```python
from build123d import *

# Parameters (mm, degrees)
SKETCH1_W           = 96.52
SKETCH1_H           = 44.45
BOSS_EXTRUDE1_DEPTH = 6.096
CUT_EXTRUDE1_REACH  = 108.961
SKETCH2_R           = 11.50874
CUT_EXTRUDE2_REACH  = 108.438
SKETCH3_R           = 3.3782
CUT_EXTRUDE3_REACH  = 108.961
SKETCH7_W           = 12.7635
SKETCH7_H           = 12.192
CUT_EXTRUDE5_DEPTH  = 104.946532487
FILLET1_R           = 11.43


with BuildPart() as part:
    # Sketch1 → Boss-Extrude1 (new, symmetric)
    with BuildSketch(Plane.XY):
        with Locations((48.26, -22.225)):
            Rectangle(SKETCH1_W, SKETCH1_H)
    extrude(amount=BOSS_EXTRUDE1_DEPTH, both=True)

    # Sketch2 → Cut-Extrude1 (cut, up to next)
    with BuildSketch(Plane.XY.offset(6.096), mode=Mode.PRIVATE) as cut_extrude1_sk1:
        with Locations((22.225, -22.225)):
            Circle(SKETCH2_R)
    cut_extrude1_tool1 = extrude(cut_extrude1_sk1.sketch, amount=-CUT_EXTRUDE1_REACH, mode=Mode.PRIVATE) & part.part
    add(cut_extrude1_tool1.solids().sort_by_distance((22.225, -22.225, 6.096))[0], mode=Mode.SUBTRACT)

    # Sketch3 → Cut-Extrude2 (cut, up to next)
    with BuildSketch(Plane(origin=(0, 0, 0), x_dir=(1, 0, 0), z_dir=(0, 1, 0)), mode=Mode.PRIVATE) as cut_extrude2_sk1:
        with Locations(Location((77.4065, -0.254, 0), (0, 0, 270))):
            Circle(SKETCH3_R)
    cut_extrude2_tool1 = extrude(cut_extrude2_sk1.sketch, amount=-CUT_EXTRUDE2_REACH, mode=Mode.PRIVATE) & part.part
    add(cut_extrude2_tool1.solids().sort_by_distance((77.4065, 0, 0.254))[0], mode=Mode.SUBTRACT)

    # Sketch4 → Cut-Extrude3 (cut, up to next)
    with BuildSketch(Plane.XY.offset(6.096), mode=Mode.PRIVATE) as cut_extrude3_sk1:
        with BuildLine():
            Line((48.895, 6.35), (96.52, 6.35))
            ThreePointArc((96.52, 6.35), (102.87, 0), (96.52, -6.35))
            Line((96.52, -6.35), (48.895, -6.35))
            ThreePointArc((48.895, -6.35), (42.545, 0), (48.895, 6.35))
        make_face()
    cut_extrude3_tool1 = extrude(cut_extrude3_sk1.sketch, amount=-CUT_EXTRUDE3_REACH, mode=Mode.PRIVATE) & part.part
    # Sketch4 → Cut-Extrude3 (cut, up to next)
    with BuildSketch(Plane.XY.offset(6.096), mode=Mode.PRIVATE) as cut_extrude3_sk2:
        with BuildLine():
            Line((45.72, -34.925), (45.72, -44.45))
            Line((45.72, -44.45), (55.245, -44.45))
            Line((55.245, -44.45), (96.52, -44.45))
            ThreePointArc((96.52, -44.45), (106.045, -34.925), (96.52, -25.4))
            Line((96.52, -25.4), (55.245, -25.4))
            ThreePointArc((55.245, -25.4), (48.509807909, -28.189807909), (45.72, -34.925))
        make_face()
    cut_extrude3_tool2 = extrude(cut_extrude3_sk2.sketch, amount=-CUT_EXTRUDE3_REACH, mode=Mode.PRIVATE) & part.part
    add(cut_extrude3_tool1.solids().sort_by_distance((72.7075, 0, 6.096))[0], mode=Mode.SUBTRACT)
    add(cut_extrude3_tool2.solids().sort_by_distance((75.382091, -35.05704, 6.096))[0], mode=Mode.SUBTRACT)

    # Sketch7 → Cut-Extrude5 (cut, through all)
    with BuildSketch(Plane(origin=(0, -6.35, 0), x_dir=(1, 0, 0), z_dir=(0, 1, 0))):
        with Locations((90.13825, 0)):
            Rectangle(SKETCH7_W, SKETCH7_H)
    extrude(amount=-CUT_EXTRUDE5_DEPTH, mode=Mode.SUBTRACT)

    # Fillet1
    fillet1_edges = [part.edges().sort_by_distance(p)[0] for p in [
        (42.545, 0, 0),
        (45.72, -44.45, 0),
        (0, -44.45, 0),
        (0, 0, 0),
    ]]
    fillet(fillet1_edges, radius=FILLET1_R)


solid = part.part
```
Geometry: final body of the model. Coordinates: model frame, mm. A direction names the side the tool comes from. Give positions to 0.01 mm unless a question says otherwise; leave off trailing zeros. Write each loop counter-clockwise with the first axis right and the second up, starting at its lowest first coordinate (ties: lowest second). Pieces come first, ordered by that corner, then holes.
1. Section query B-B, the plane x = 20. Return loops of the section in (y, z).
2. Section query C-C, the plane z = 0.5. Count the separate pieces of the cut face and the enclosed holes in it, then the cut area to 3 significant figures.
3. Section query D-D, the plane y = -32. Return loops of the section in (x, z).
4. Reachability of faces 4 (the flat face through (23, 0, 0)), 5 (the flat face through (67, -6.35, 0)), 6 (the flat face through (70, -25.4, 0)) from +Z, -Z, +X, -X, +Y, -Y: full face, straight path, thin tool, end or side. Return the list, or none.
5. Line query: probe 1 along Y at (x, z) = (64, 0.5); probe 2 along X at (y, z) = (-13, 2.5); probe 3 along Y at (x, z) = (26, 1.75). Output: solid intervals per line, ascending.
6. Pin query (flat end, axial travel): P1, Ø6, axis at x = 74.5, z = -0.5, coming from the +Y side; P2, Ø3.5, axis at x = 65, z = 1, coming from the -Y side; P3, Ø3, axis at y = -9, z = 4.5, coming from the -X side. Return the tip coordinate at first contact, or that it passes through.
7. Draft query along Z for faces 1 (the cylindrical face through (74.41, -15.74, 1.81)), 2 (the cylindrical face through (3.259, -3.437, -0.085)), 3 (the flat face through (41, -22, -6.096)). Return one class per face: released by +Z, released by -Z, zero draft, split by the parting line, or undercut.
8. Section query A-A, the plane y = -16. Return loops of the section in (x, z).
Computed:
1. outline: (-44.45, -6.1) - (-33.52, -6.1) - (-33.52, 6.1) - (-44.45, 6.1) - close; (-10.93, -6.1) - (0, -6.1) - (0, 6.1) - (-10.93, 6.1) - close
2. separate pieces: 2
2. enclosed holes: 1
2. area: 2,130 mm2
3. outline: (0, -6.1) - (16.15, -6.1) - (16.15, 6.1) - (0, 6.1) - close; (28.3, -6.1) - (46.18, -6.1) - (46.18, 6.1) - (28.3, 6.1) - close
4. face 4: +Z, -Z, +X, -X, +Y
4. face 5: +Z, -Z, +X, +Y
4. face 6: +Z, -Z, +X, -Y
5. probe 1: y = -25.4 to -6.35
5. probe 2: x = 0 to 15.34, 29.11 to 74.88, 79.93 to 83.76
5. probe 3: y = -44.45 to -33.1, -11.35 to 0
6. P1: stops at y = -6.35
6. P2: stops at y = -25.4
6. P3: stops at x = 0.04
7. face 1: undercut
7. face 2: zero draft
7. face 3: released by -Z
8. outline: (0, -6.1) - (12.55, -6.1) - (12.55, 6.1) - (0, 6.1) - close; (31.9, -6.1) - (83.76, -6.1) - (83.76, 6.1) - (31.9, 6.1) - close; hole circle Ø6.76 at (77.41, 0.25)
